from build123d import *

# Parameters (mm, degrees)
BOSS_EXTRUDE1_DEPTH = 3
SKETCH2_R           = 3
SKETCH2_R_2         = 1.3
CUT_EXTRUDE1_DEPTH  = 47.16592358
SKETCH3_W           = 12
SKETCH3_H           = 38.3
CUT_EXTRUDE2_DEPTH  = 1
SKETCH4_W           = 12
SKETCH4_H           = 3
CUT_EXTRUDE3_DEPTH  = 47.111739286
CHAMFER1_SIZE       = 3
CUT_EXTRUDE4_DEPTH  = 47.16592358
CHAMFER2_SIZE       = 1


with BuildPart() as part:
    # Sketch1 → Boss-Extrude1 (new body)
    with BuildSketch(Plane(origin=(0, 0, 0), x_dir=(1, 0, 0), z_dir=(0, 1, 0))):
        Polygon((0, 23.05), (0, -23.05), (-12.5, -23.05), (-12.5, -35.55), (29.3, -35.55), (29.3, -21.55), (15.3, -21.55), (15.3, 21.55), (29.3, 21.55), (29.3, 35.55), (-12.5, 35.55), (-12.5, 23.05), align=None)
    extrude(amount=BOSS_EXTRUDE1_DEPTH)

    # Sketch2 → Cut-Extrude1 (cut, through all)
    with BuildSketch(Plane(origin=(0, 3, 0), x_dir=(1, 0, 0), z_dir=(0, 1, 0))):
        with Locations(Location((-6.25, 29.3, 0), (0, 0, 270))):
            Circle(SKETCH2_R)
        with Locations(Location((-6.25, -29.3, 0), (0, 0, 270))):
            Circle(SKETCH2_R)
        with Locations(Location((22.3, -28.55, 0), (0, 0, 270))):
            Circle(SKETCH2_R_2)
        with Locations(Location((22.3, 28.55, 0), (0, 0, 270))):
            Circle(SKETCH2_R_2)
    extrude(amount=-CUT_EXTRUDE1_DEPTH, mode=Mode.SUBTRACT)

    # Sketch3 → Cut-Extrude2 (cut)
    with BuildSketch(Plane(origin=(0, 3, 0), x_dir=(1, 0, 0), z_dir=(0, 1, 0))):
        with Locations((7.65, 0)):
            Rectangle(SKETCH3_W, SKETCH3_H)
    extrude(amount=-CUT_EXTRUDE2_DEPTH, mode=Mode.SUBTRACT)

    # Sketch4 → Cut-Extrude3 (cut, through all)
    with BuildSketch(Plane(origin=(0, 2, 0), x_dir=(1, 0, 0), z_dir=(0, 1, 0))):
        with Locations((7.65, -17.65)):
            Rectangle(SKETCH4_W, SKETCH4_H)
    extrude(amount=-CUT_EXTRUDE3_DEPTH, mode=Mode.SUBTRACT)

    # Chamfer1
    chamfer1_edges = [part.edges().sort_by_distance(p)[0] for p in [
        (0, 1.5, 23.05),
        (0, 1.5, -23.05),
    ]]
    chamfer(chamfer1_edges, length=CHAMFER1_SIZE)

    # Sketch5 → Cut-Extrude4 (cut, through all)
    with BuildSketch(Plane(origin=(0, 3, 0), x_dir=(1, 0, 0), z_dir=(0, 1, 0))):
        Polygon((4.037233657, -35.55), (6.218616828, -39.328266484), (10.581383172, -39.328266484), (12.762766343, -35.55), (10.581383172, -31.771733516), (6.218616828, -31.771733516), align=None)
        Polygon((4.037233657, 35.55), (6.218616828, 31.771733516), (10.581383172, 31.771733516), (12.762766343, 35.55), (10.581383172, 39.328266484), (6.218616828, 39.328266484), align=None)
    extrude(amount=-CUT_EXTRUDE4_DEPTH, mode=Mode.SUBTRACT)

    # Chamfer2
    chamfer2_edges = [part.edges().sort_by_distance(p)[0] for p in [
        (-12.5, 1.5, -23.05),
        (-12.5, 1.5, -35.55),
        (29.3, 1.5, -35.55),
        (29.3, 1.5, -21.55),
        (29.3, 1.5, 21.55),
        (29.3, 1.5, 35.55),
        (-12.5, 1.5, 35.55),
        (-12.5, 1.5, 23.05),
    ]]
    chamfer(chamfer2_edges, length=CHAMFER2_SIZE)


solid = part.part
Can you work these out from the model? Positions are in its coordinate system, mm. A direction names the side the tool comes from. Give positions to 0.01 mm unless a question says otherwise; leave off trailing zeros. Order: outer loops, then holes, each group sorted by start corner. A loop starts at its lowest first (then second) coordinate and runs counter-clockwise, first axis right, second up. Notation, with made-up numbers: M -19,14.5 L 21,14.5 A32 cw 21,50.5 Z; hole C -1,15.5 d3. An arc over 180 degrees is marked long. Use one line per item in the form item = value.
Item 1: Will these pins go through, and if not, where does the flat tip stop? pin 1 Ø1.5 at (x, y) = (9, 2.5) entering from -Z; pin 2 Ø1.6 at (x, z) = (22.3, 28.55) entering from -Y; pin 3 Ø0.8 at (x, y) = (5.5, 2.5) entering from +Z; pin 4 Ø0.9 at (y, z) = (1, 2) entering from -X.
Values follow:
pin_1 = -31.77
pin_2 = through
pin_3 = 33.71
pin_4 = 0
Item 2: If I drill on line 1 along X through (y, z) = (2.45, 8); line 2 along X through (y, z) = (0.75, -29.3); line 3 along Z through (x, y) = (-1.5, 1.95), over which ranges is the centre line in solid material (lowest first)? Write a range as [from, to].
Values follow:
line_1 = [0, 1.65], [13.65, 15.3]
line_2 = [-12.5, -9.25], [-3.25, 21.24], [23.36, 29.3]
line_3 = [-35.55, -21.55], [21.55, 35.55]
Item 3: If we section it at A-A, the plane x = -6.25: Write out the boundary of the cut face in (y, z).
Values follow:
outline = M 0,-35.55 L 3,-35.55 L 3,-32.3 L 0,-32.3 Z; M 0,-26.3 L 3,-26.3 L 3,-23.05 L 0,-23.05 Z; M 0,23.05 L 3,23.05 L 3,26.3 L 0,26.3 Z; M 0,32.3 L 3,32.3 L 3,35.55 L 0,35.55 Z
Item 4: If we section it at C-C, the plane z = 28.55: Write out the boundary of the cut face in (x, y).
Values follow:
outline = M -12.5,0 L -9.15,0 L -9.15,3 L -12.5,3 Z; M -3.35,0 L 21,0 L 21,3 L -3.35,3 Z; M 23.6,0 L 29.3,0 L 29.3,3 L 23.6,3 Z
Item 5: Thinking about a two-plate mould opening in Z: for faces 1 (the flat face through (-7, 1, 23.05)), 2 (the flat face through (11.69, 1.52, 33.69)), 3 (the flat face through (11.657, 1.521, -33.634)), 4 (the flat face through (29.3, 1, -28)), which applies, pulls with the +Z half, pulls with the -Z half, needs draft (parallel to the pull), parting line crosses it, or undercut?
Values follow:
face_1 = undercut
face_2 = pulls with the +Z half
face_3 = pulls with the -Z half
face_4 = needs draft
Item 6: For faces 5 (the flat face through (8, 2, 31.772)), 6 (the flat face through (13.65, 2.2, 4.5)), 7 (the flat face through (-4, 1, 35.55)), 8 (the flat face through (15.3, 1, 0)), 9 (the flat face through (-1.52, 1.48, 21.57)), which set-ups out of +Z, -Z, +X, -X, +Y, -Y let a thin tool reach every point of the face, with its end or its side?
Values follow:
face_5 = +Z, +Y, -Y
face_6 = +Y
face_7 = +Z, +X, -X, +Y, -Y
face_8 = +X, +Y, -Y
face_9 = -X, +Y, -Y
Item 7: If we section it at B-B, the plane z = 1.5: Write out the boundary of the cut face in (x, y), and give its area (3 significant figures).
Values follow:
outline = M 0,0 L 15.3,0 L 15.3,3 L 13.65,3 L 13.65,2 L 1.65,2 L 1.65,3 L 0,3 Z
area = 33.9 mm^2
